Autodesk Inventor part; units mm, degrees
ref_plane "YZ Plane" through (0, 0, 0) normal (1, 0, 0) x (0, 1, 0)
ref_plane "XZ Plane" through (0, 0, 0) normal (0, 1, 0) x (-1, 0, 0)
ref_plane "XY Plane" through (0, 0, 0) normal (0, 0, 1) x (1, 0, 0)
sketch "Sketch1" plane through (0, 0, 0) normal (0, 1, 0) x (-1, 0, 0)
  line L0 (10, 10) -> (-10, 10)
  line L1 (-10, 10) -> (-10, -10)
  line L2 (-10, -10) -> (10, -10)
  line L3 (10, -10) -> (10, 10)
  line L4 (10, 10) -> (-10, -10) construction
  line L5 (-10, 10) -> (10, -10) construction
  point P0 (0, 0)
  dimension "d0" = 20
  dimension "d1" = 20
extrude "Extrusion1" add sketch "Sketch1" along normal blind 5
sketch "Sketch2" plane through (0, 5, 0) normal (0, 1, 0) x (1, 0, 0)
  circle A0 centre (0, 0) radius 7.4
  dimension "d4" = 14.8
extrude "Extrusion2" add sketch "Sketch2" along normal blind 10
sketch "Sketch3" plane through (-10, 0, 10) normal (0, 0, 1) x (1, 0, 0)
  circle A0 centre (10, 10) radius 1.55
  line L0 (0, 5) -> (20, 5)
  point P0 (10, 0)
  dimension "d7" = 3.1
  dimension "d8" = 5
extrude "Extrusion3" cut sketch "Sketch3" against normal through all
fillet "Fillet1" radius 2 5 edges at (10, 2.5, 10) (10, 2.5, -10) (0, 0, 10) (10, 0, 0) (0, 0, -10)
properties part number "finger2+" material "ABS Plastic"
Design review of the part built by this model. Coordinates are the model's own, in mm. A direction names the side the tool comes from. Coordinates: 2 decimals unless noted, no trailing zeros. Write each loop counter-clockwise with the first axis right and the second up, starting at its lowest first coordinate (ties: lowest second). Pieces come first, ordered by that corner, then holes. Notation, with made-up numbers: (4.5, 87.25) -> (12.5, 87.25) arc R33 ccw to (12.5, 120.25) -> close; hole circle Ø2 at (11.25, 61). An arc over 180 degrees is marked (long way). Write each question's results on one line, items separated by ' | '. Start each with the question number.
(1) For line 1 along X through (y, z) = (10, 0); line 2 along Y through (x, z) = (0, 1.5); line 3 along Y through (x, z) = (-7, -6.5), list the stretches that pass through material, from the lowest coordinate up. Write a range as from..to.
(2) Tool access review of faces 4 (the face through (3.415, 9.93, -6.565)), 5 (the face through (-0.87, 0.6, 9.43)): name each direction out of +Z, -Z, +X, -X, +Y, -Y from which nothing blocks a thin tool from reaching the whole face with its end or side.
(3) Take a section at C-C on y = 6.25. Write out the cut boundary in (x, z), and give its area (3 significant figures).
(4) The part is to be moulded in two halves that separate along X. For faces 1 (the face through (-0.336, 8.487, 0.104)), 2 (the face through (-4, 5, 7)), 3 (the face through (9.43, 0.6, -0.11)), say which applies: pulls with the +X half, pulls with the -X half, needs draft (parallel to the pull), parting line crosses it, or undercut.
(5) Take a section at A-A on x = 0. Write out the cut boundary in (y, z), and give its area (3 significant figures).
(6) Clearance check with flat-ended pins moving along their axes: P1, Ø8, axis at y = 10, z = 3.5, coming from the +X side; P2, Ø2, axis at x = -6, z = -6, coming from the +Y side; P3, Ø2.5, axis at x = 0, y = 10, coming from the -Z side; P4, Ø1.5, axis at x = -2, y = 7, coming from the +Z side. State where each tip first meets the part, or that it passes through.
(7) Take a section at B-B on z = 0. Write out the cut boundary in (x, y), and give its area (3 significant figures).
(8) Take a section at D-D on y = 10. Write out the cut boundary in (x, z), and give its area (3 significant figures).
Results found:
1) line 1: x = -7.4..-1.55, 1.55..7.4 | line 2: y = 0..8.45, 11.55..15 | line 3: y = 0..5
2) face 4: +Y | face 5: +Z, +X, -X, -Y
3) outline: circle Ø14.8 at (0, 0) | area: 172 mm2
4) face 1: undercut | face 2: needs draft | face 3: pulls with the +X half
5) outline: (0, -8) arc R2 ccw to (2, -10) -> (5, -10) -> (5, -7.4) -> (8.45, -7.4) -> (8.45, 7.4) -> (5, 7.4) -> (5, 10) -> (2, 10) arc R2 ccw to (0, 8) -> close; (11.55, -7.4) -> (15, -7.4) -> (15, 7.4) -> (11.55, 7.4) -> close | area: 200 mm2
6) P1: stops at x = 7.4 | P2: stops at y = 5 | P3: passes through | P4: stops at z = 7.29
7) outline: (-10, 0) -> (8, 0) arc R2 ccw to (10, 2) -> (10, 5) -> (7.4, 5) -> (7.4, 15) -> (-7.4, 15) -> (-7.4, 5) -> (-10, 5) -> close; hole circle Ø3.1 at (0, 10) | area: 240 mm2
8) outline: (-1.55, -7.24) -> (-1.55, 7.24) arc R7.4 ccw to start; (1.55, -7.24) arc R7.4 ccw to (1.55, 7.24) -> close | area: 126 mm2
